Part model, mm, in its own coordinate system. A direction names the side the tool comes from. Give positions to 0.01 mm unless a question says otherwise; leave off trailing zeros. Order: outer loops, then holes, each group sorted by start corner. A loop starts at its lowest first (then second) coordinate and runs counter-clockwise, first axis right, second up. Notation, with made-up numbers: (81, 78.25) - (129, 78.25) arc R13 ccw to (129, 98.25) - close; hole circle Ø10 at (27, -13.5). An arc over 180 degrees is marked (long way). One line per item, written item: value.
```python
from build123d import *

# Parameters (mm, degrees)
EXTRUDE_1_DEPTH      = 45
EXTRUDE_1_DEPTH_BACK = 16
SKETCH_1_R           = 4
SKETCH_3_R           = 1.5
CUT_EXTRUDE_1_DEPTH  = 10
CHAMFER_1_SIZE       = 1
EXTRUDE_START        = -39
SKETCH_5_R           = 5
EXTRUDE_3_DEPTH      = 7
SKETCH_8_R           = 1.5
CUT_EXTRUDE_2_DEPTH  = 10
CHAMFER_2_SIZE       = 1


with BuildPart() as part:
    # Sketch 1 → Extrude 1 (new, two sides: drawn at the far end of the back side and taken through both)
    with BuildSketch(Plane.XY.offset(-EXTRUDE_1_DEPTH_BACK)):
        Circle(SKETCH_1_R)
    extrude(amount=EXTRUDE_1_DEPTH + EXTRUDE_1_DEPTH_BACK)

    # Sketch 3 → Cut-Extrude 1 (cut)
    with BuildSketch(Plane(origin=(0, 0, 0), x_dir=(1, 0, 0), z_dir=(0, 1, 0))):
        with Locations(Location((0, -17.5, 0), (0, 0, 270))):
            Circle(SKETCH_3_R)
    extrude(amount=-CUT_EXTRUDE_1_DEPTH, mode=Mode.SUBTRACT)

    # Chamfer 1
    chamfer_1_edges = [part.edges().sort_by_distance(p)[0] for p in [
        (-4, 0, 45),
    ]]
    chamfer(chamfer_1_edges, length=CHAMFER_1_SIZE)

    # Sketch 5 → Extrude 3 (add)
    with BuildSketch(Plane.XY.offset(45).offset(EXTRUDE_START)):
        Circle(SKETCH_5_R)
    extrude(amount=EXTRUDE_3_DEPTH)

    # Sketch 8 → Cut-Extrude 2 (cut)
    with BuildSketch(Plane(origin=(0, 0, 0), x_dir=(1, 0, 0), z_dir=(0, 1, 0))):
        with Locations(Location((0, 11, 0), (0, 0, 270))):
            Circle(SKETCH_8_R)
    extrude(amount=-CUT_EXTRUDE_2_DEPTH, mode=Mode.SUBTRACT)

    # Chamfer 2
    chamfer_2_edges = [part.edges().sort_by_distance(p)[0] for p in [
        (-4, 0, -16),
    ]]
    chamfer(chamfer_2_edges, length=CHAMFER_2_SIZE)


solid = part.part
```
1) Cut at B-B, the plane z = 8. Give the cut face in (x, y), then the cut area to 3 significant figures.
Outcome:
outline: circle Ø10 at (0, 0)
area: 78.5 mm^2
2) Cut at A-A, the plane x = 0. Give the cut face in (y, z), then the cut area to 3 significant figures.
Outcome:
outline: (-5, 6) - (-4, 6) - (-4, -9.5) - (0, -9.5) - (0, -12.5) - (-4, -12.5) - (-4, -15) - (-3, -16) - (3, -16) - (4, -15) - (4, 6) - (5, 6) - (5, 13) - (4, 13) - (4, 44) - (3, 45) - (-3, 45) - (-4, 44) - (-4, 19) - (0, 19) - (0, 16) - (-4, 16) - (-4, 13) - (-5, 13) - close
area: 476 mm^2
3) Cut at C-C, the plane y = -2. Give the number of separate pieces and of enclosed holes in the cut face, then the cut area to 3 significant figures.
Outcome:
separate pieces: 1
enclosed holes: 2
area: 422 mm^2
4) Drill centre lines: line 1 along Z through (x, y) = (0, -1.45); line 2 along Z through (x, y) = (1.25, -1); line 3 along X through (y, z) = (-2.2, -11). Where is each one in solid material? Low to high. Write a range as from..to.
Outcome:
line 1: z = -16..-12.5, -9.5..16, 19..45
line 2: z = -16..-11.83, -10.17..16.67, 18.33..45
line 3: x = -3.34..-1.5, 1.5..3.34
5) Mould opens along Z. For faces 5 (the flat face through (0, 0, 45)), 6 (the flat face through (0, 0, -16)), 7 (the flat face through (0, 0, -11)) say: released by +Z, released by -Z, zero draft, split by the parting line, or undercut.
Outcome:
face 5: released by +Z
face 6: released by -Z
face 7: undercut
6) Which spindle directions (+Z, -Z, +X, -X, +Y, -Y) get a long thin tool onto all of the face, cutting with end or side? Do faces 1 (the cylindrical face through (-1.08, -4.88, 9.45)), 2 (the cylindrical face through (2.15, 3.373, -4.647)), 3 (the cylindrical face through (2.15, 3.373, 28.283)), 4 (the cylindrical face through (-0.575, -1.973, -9.614)). Say none if no direction does.
Outcome:
face 1: +Z, -Z
face 2: -Z
face 3: +Z
face 4: -Y
7) Cut at D-D, the plane z = 0.5. Give the cut face in (x, y).
Outcome:
outline: circle Ø8 at (0, 0)
8) Pin check, flat tips, straight feed: pin 1 (2 mm diameter, centred on y = -3, z = 33.5, fed in from +X); pin 2 (6 mm diameter, centred on y = 1.5, z = 25.5, fed in from -X); pin 3 (2 mm diameter, centred on x = -3.5, z = 20, fed in from -Y). Stop position of each tip, or through.
Outcome:
pin 1: stops at x = 3.46
pin 2: stops at x = -4
pin 3: stops at y = -3.12
